Design review of the part built by this model. Coordinates are the model's own, in mm. Coordinates: 2 decimals unless noted, no trailing zeros. Write each loop counter-clockwise with the first axis right and the second up, starting at its lowest first coordinate (ties: lowest second). Pieces come first, ordered by that corner, then holes. Notation, with made-up numbers: M 5.25,63 L 35.25,63 A32 ccw 35.25,90 Z; hole C 67.25,11.25 d4. An arc over 180 degrees is marked long. Write item = value, one per line.
```python
from build123d import *

# Parameters (mm, degrees)
SKETCH1_W               = 195
SKETCH1_H               = 180
BOSS_EXTRUDE1_DEPTH     = 3.175
SKETCH2_W               = 65
SKETCH2_H               = 6.35
BOSS_EXTRUDE2_DEPTH     = 6.35
LPATTERN1_COUNT         = 2
LPATTERN1_PITCH         = 130
MIRROR1_COPY_1_SKETCH_W = 65
MIRROR1_COPY_1_SKETCH_H = 6.35
MIRROR1_COPY_1_DEPTH    = 6.35
SKETCH3_W               = 6.35
SKETCH3_H               = 65
BOSS_EXTRUDE3_DEPTH     = 6.35
SKETCH4_R               = 2
CUT_EXTRUDE1_DEPTH      = 7.35
FILLET1_R               = 1
CUT_EXTRUDE2_DEPTH      = 7.35
SKETCH6_R               = 2
CUT_EXTRUDE3_DEPTH      = 7.35
FILLET2_R               = 1
FILLET3_R               = 5


with BuildPart() as part:
    # Sketch1 → Boss-Extrude1 (new body, symmetric)
    with BuildSketch(Plane(origin=(0, 0, 0), x_dir=(1, 0, 0), z_dir=(0, 1, 0))):
        with Locations((97.5, 90)):
            Rectangle(SKETCH1_W, SKETCH1_H)
    extrude(amount=BOSS_EXTRUDE1_DEPTH, both=True)

    # Sketch2 → Boss-Extrude2 (add)
    with BuildSketch(Plane(origin=(0, 3.175, 0), x_dir=(1, 0, 0), z_dir=(0, 1, 0))):
        with Locations((162.5, -3.175)):
            Rectangle(SKETCH2_W, SKETCH2_H)
    boss_extrude2 = extrude(amount=-BOSS_EXTRUDE2_DEPTH)

    # LPattern1: Boss-Extrude2 ×2
    with Locations(*[(-i * LPATTERN1_PITCH, 0, 0) for i in range(1, LPATTERN1_COUNT)]):
        add(boss_extrude2)

    # Mirror1: Boss-Extrude2 across plane
    add(boss_extrude2.mirror(Plane.XY.offset(-90)))

    # Mirror1 copy 1 sketch → Mirror1 copy 1 (add)
    with BuildSketch(Plane(origin=(-130, 3.175, -180), x_dir=(1, 0, 0), z_dir=(0, 1, 0))):
        with Locations((162.5, 3.175)):
            Rectangle(MIRROR1_COPY_1_SKETCH_W, MIRROR1_COPY_1_SKETCH_H)
    extrude(amount=-MIRROR1_COPY_1_DEPTH)

    # Sketch3 → Boss-Extrude3 (add)
    with BuildSketch(Plane(origin=(0, 3.175, 0), x_dir=(1, 0, 0), z_dir=(0, 1, 0))):
        with Locations((-3.175, 137.5)):
            Rectangle(SKETCH3_W, SKETCH3_H)
        with Locations((-3.175, 42.5)):
            Rectangle(SKETCH3_W, SKETCH3_H)
    extrude(amount=-BOSS_EXTRUDE3_DEPTH)

    # Sketch4 → Cut-Extrude1 (cut, through all)
    with BuildSketch(Plane(origin=(0, 3.175, 0), x_dir=(1, 0, 0), z_dir=(0, 1, 0))):
        with Locations((65, 0)):
            Circle(SKETCH4_R)
        with Locations((130, 0)):
            Circle(SKETCH4_R)
    extrude(amount=-CUT_EXTRUDE1_DEPTH, mode=Mode.SUBTRACT)

    # Fillet1
    fillet1_edges = [part.edges().sort_by_distance(p)[0] for p in [
        (130, 0, 6.35),
        (65, 0, 6.35),
    ]]
    fillet(fillet1_edges, radius=FILLET1_R)

    # Sketch5 → Cut-Extrude2 (cut, through all)
    with BuildSketch(Plane(origin=(0, 3.175, 0), x_dir=(1, 0, 0), z_dir=(0, 1, 0))):
        with BuildLine():
            Line((130, -2.828427125), (130, -5.35))
            ThreePointArc((130, -5.35), (130.292893219, -6.057106781), (131, -6.35))
            Line((131, -6.35), (64, -6.35))
            ThreePointArc((64, -6.35), (64.707106781, -6.057106781), (65, -5.35))
            Line((65, -5.35), (65, -2.828427125))
            ThreePointArc((65, -2.828427125), (64.816496581, -2.251076856), (64.333333333, -1.885618083))
            ThreePointArc((64.333333333, -1.885618083), (63.585786438, 1.414213562), (66.885618083, 0.666666667))
            ThreePointArc((66.885618083, 0.666666667), (67.251076856, 0.183503419), (67.828427125, 0))
            Line((67.828427125, 0), (127.171572875, 0))
            ThreePointArc((127.171572875, 0), (127.748923144, 0.183503419), (128.114381917, 0.666666667))
            ThreePointArc((128.114381917, 0.666666667), (131.414213562, 1.414213562), (130.666666667, -1.885618083))
            ThreePointArc((130.666666667, -1.885618083), (130.183503419, -2.251076856), (130, -2.828427125))
        make_face()
    cut_extrude2 = extrude(amount=-CUT_EXTRUDE2_DEPTH, mode=Mode.SUBTRACT)

    # Mirror3: Cut-Extrude2 across plane
    add(cut_extrude2.mirror(Plane.XY.offset(-90)), mode=Mode.SUBTRACT)

    # Sketch6 → Cut-Extrude3 (cut, through all)
    with BuildSketch(Plane(origin=(0, 3.175, 0), x_dir=(1, 0, 0), z_dir=(0, 1, 0))):
        with Locations((0, 105)):
            Circle(SKETCH6_R)
        with Locations((0, 75)):
            Circle(SKETCH6_R)
    extrude(amount=-CUT_EXTRUDE3_DEPTH, mode=Mode.SUBTRACT)

    # Fillet2
    fillet2_edges = [part.edges().sort_by_distance(p)[0] for p in [
        (-2, 0, -75),
        (-2, 0, -105),
        (0, 0, -103),
        (0, 0, -77),
        (-6.35, 0, -105),
        (-6.35, 0, -75),
    ]]
    fillet(fillet2_edges, radius=FILLET2_R)

    # Fillet3
    fillet3_edges = [part.edges().sort_by_distance(p)[0] for p in [
        (195, 0, 6.35),
        (0, 0, 6.35),
        (195, 0, -186.35),
        (0, 0, -186.35),
        (-6.35, 0, -170),
        (-6.35, 0, -10),
    ]]
    fillet(fillet3_edges, radius=FILLET3_R)


solid = part.part
```
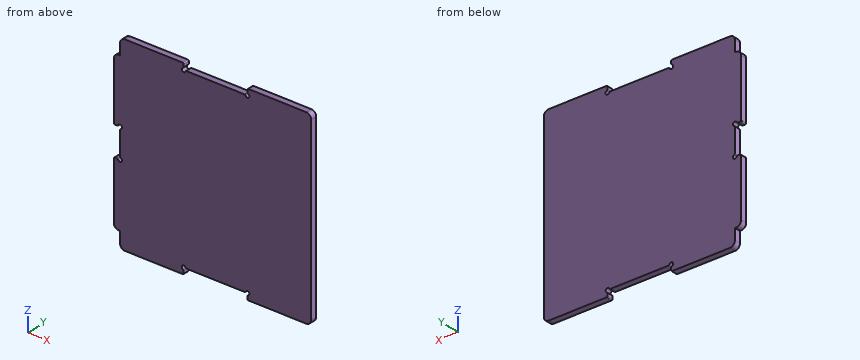
Q1. For P1, Ø1.5, axis at x = -1, y = -0.5, coming from the -Z side; P2, Ø0.8, axis at y = 1, z = 4.5, coming from the +X side; P3, Ø2.5, axis at x = 0, z = -105, coming from the +Y side; P4, Ø1.9, axis at x = 92.5, y = -1.5, coming from the -Z side, all flat-tipped, find the tip position at first contact; note any pin that passes through.
Check result:
P1 = -170
P2 = 194.18
P3 = through
P4 = -180
Q2. Wall thickness on line 1 (Z direction, x = 92, y = 1.25): over which ranges is the line inside the solid? List them lowest first.
Check result:
line_1 = -180 to 0
Q3. Consider section A-A, the plane z = -80.5. State the section outline as (x, y) points (3 decimals), and give its area (3 significant figures).
Check result:
outline = M 0,-3.175 L 195,-3.175 L 195,3.175 L 0,3.175 Z
area = 1,240 mm²
